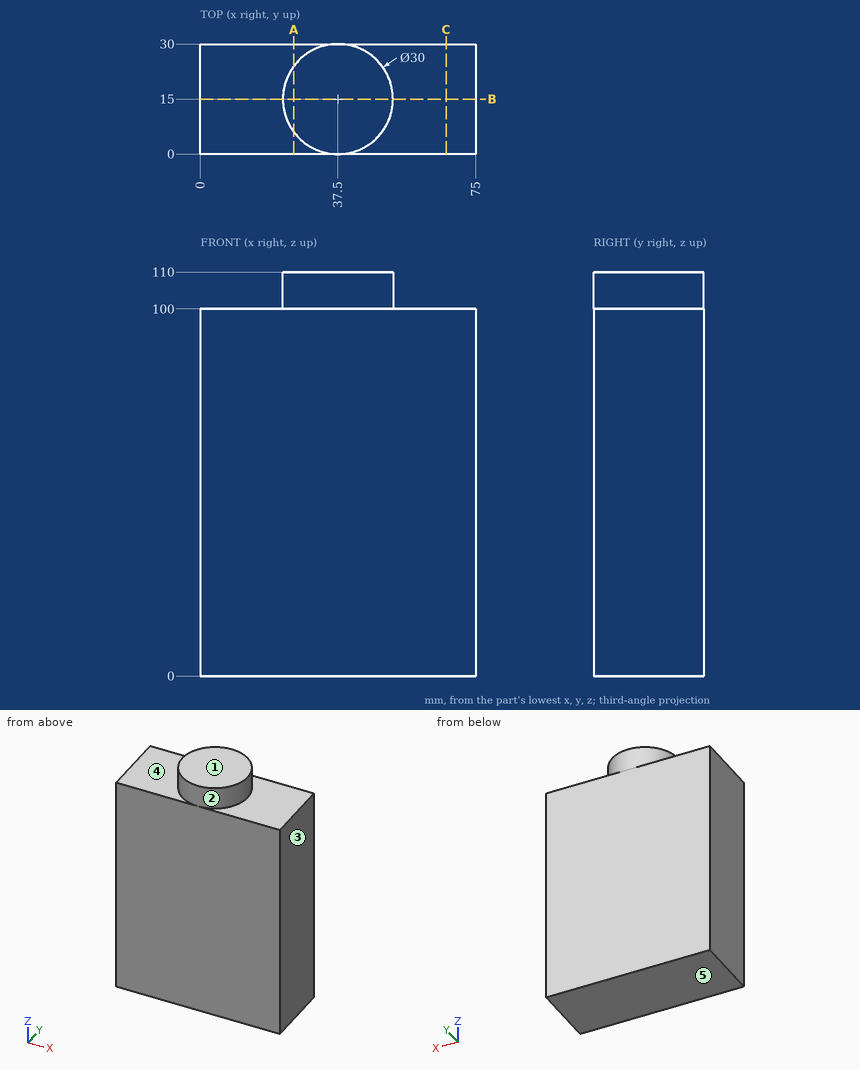
Could you check a few things on this drawing? It's one solid part, dimensions in mm from its lowest x, y, z. A direction names the side the tool comes from. Coordinates: 2 decimals unless noted, no trailing zeros. Order: outer loops, then holes, each group sorted by start corner. A loop starts at its lowest first (then second) coordinate and runs counter-clockwise, first axis right, second up. Notation, with made-up numbers: (46.5, 20.25) -> (104.5, 20.25) arc R24 ccw to (104.5, 30.25) -> close; hole circle Ø5 at (7, 12.25). An arc over 180 degrees is marked (long way). One line per item, written item: value. Start each with the question number.
1) Imagine slicing it at C-C on x = 67. List the corners of the cut face in (y, z) for me.
2) Imagine slicing it at B-B on y = 15. List the corners of the cut face in (x, z) for me.
3) We'd pull the mould along Z, two halves only. Please class the marked faces 3, 4 and 5: +Z half, -Z half, draft (parallel to the pull), parting line (faces both ways), or undercut.
4) Which directions (+Z, -Z, +X, -X, +Y, -Y) give clear straight access to the entire face, cutting with the end or side of a thin tool? Please do the marked faces 1 and 2.
5) I'm going to push a flat-ended pin straight in: pin 1 (6 mm diameter, centred on x = 8.5, y = 7, fed in from +Z). Where does the tip first touch, or does it pass through?
6) If I drill on L1, parallel to Z at x = 65.5, y = 23; L2, parallel to Y at x = 31, z = 105; L3, parallel to X at y = 8.75, z = 103, over which ranges is the centre line in solid material (lowest first)? Write a range as [from, to].
7) Imagine slicing it at A-A on x = 25.5. List the corners of the cut face in (y, z) for me, plus the area to 3 significant figures.
Answer list:
1. outline: (0, 0) -> (30, 0) -> (30, 100) -> (0, 100) -> close
2. outline: (0, 0) -> (75, 0) -> (75, 100) -> (52.5, 100) -> (52.5, 110) -> (22.5, 110) -> (22.5, 100) -> (0, 100) -> close
3. face 3: draft
3. face 4: +Z half
3. face 5: -Z half
4. face 1: +Z, +X, -X, +Y, -Y
4. face 2: +Z
5. pin 1: stops at z = 100
6. L1: z = [0, 100]
6. L2: y = [1.48, 28.52]
6. L3: x = [23.86, 51.14]
7. outline: (0, 0) -> (30, 0) -> (30, 100) -> (24, 100) -> (24, 110) -> (6, 110) -> (6, 100) -> (0, 100) -> close
7. area: 3,180 mm2
